```python
from build123d import *

# Parameters (mm, degrees)
F2_SIZE = 1


with BuildPart() as f1:
    # F0 (on Right) → F1 (revolve)
    with BuildSketch(Plane.YZ):
        Polygon((-16, 4.175502), (-20, 4.175502), (-20, -7.824498), (-16, -7.824498), (-16, -1.824498), (0, -1.824498), (0, 0.175502), (-16, 0.175502), align=None)
    revolve(axis=Axis((0, 0, -1.638931), (0, 0, -1)))

    # F2
    f2_edges = [f1.edges().sort_by_distance(p)[0] for p in [
        (0, 16, 4.175502),
        (0, 20, 4.175502),
        (0, 20, -7.824498),
        (0, 16, -7.824498),
    ]]
    chamfer(f2_edges, length=F2_SIZE)


solid = f1.part
```
CAD build for the part. Positions are in the model's coordinates, mm. A direction names the side the tool comes from. Round coordinates to 2 decimals unless told otherwise and drop trailing zeros. Loops run counter-clockwise (first coordinate to the right, second up) from the corner with the lowest first, then second, coordinate; pieces in that order, holes last. Notation, with made-up numbers: M -8.5,-28.5 L -1.5,-28.5 A31 ccw -1.5,3.5 Z; hole C 16,89.25 d5. An arc over 180 degrees is marked long. Return JSON: item names as keys, results as strings. Group by question number.
(1) Tool access for faces 1 (the cylindrical face through (15.62, 3.47, -4.29)), 2 (the flat face through (0, 0, 0.176)), 3 (the flat face through (10, 14, -7.824)): list every direction of +Z, -Z, +X, -X, +Y, -Y with a clear straight run to the whole face (end or side of a thin tool).
(2) Wall check: probe 1 along X at (y, z) = (0, 2.5); probe 2 along Z at (x, y) = (-6.5, 7). Give the ranges that are in metal, low to high. Write a range as [from, to].
(3) Mould opens along X. For faces 4 (the flat face through (10, -14, 4.176)), 5 (the cylindrical face through (19.524, 4.336, -1.894)), 6 (the flat face through (0, 0, -1.824)) say: +X half, -X half, draft (parallel to the pull), parting line (faces both ways), or undercut.
(4) Drop flat-ended pins along their axis: P1, Ø2, axis at y = -1, z = 2.5, coming from the +X side; P2, Ø12, axis at x = -6, y = 13.5, coming from the +Z side; P3, Ø3, axis at x = -6.5, z = -2, coming from the +Y side; P4, Ø3, axis at x = 3.5, z = -0.5, coming from the -Y side. Give the stop position or say it passes through.
(5) Saw through at C-C, the plane z = -5.5. List the corners of the cut face in (x, y), and give its area (3 significant figures).
(6) Saw through at A-A, the plane x = 0. List the corners of the cut face in (y, z), and give its area (3 significant figures).
(7) Saw through at D-D, the plane z = -0.5. List the corners of the cut face in (x, y), and give its area (3 significant figures).
Answer list:
{
 "1": {"face 1": "-Z", "face 2": "+Z", "face 3": "-Z, +X, -X, +Y, -Y"},
 "2": {"probe 1": "[-20, -16], [16, 20]", "probe 2": "[-1.82, 0.18]"},
 "3": {"face 4": "draft", "face 5": "parting line", "face 6": "undercut"},
 "4": {"P1": "x = 20", "P2": "z = 4.18", "P3": "y = 19.36", "P4": "y = -19.9"},
 "5": {"outline": "C 0,0 d40; hole C 0,0 d32", "area": "452 mm2"},
 "6": {"outline": "M -20,-6.82 L -19,-7.82 L -17,-7.82 L -16,-6.82 L -16,-1.82 L 16,-1.82 L 16,-6.82 L 17,-7.82 L 19,-7.82 L 20,-6.82 L 20,3.18 L 19,4.18 L 17,4.18 L 16,3.18 L 16,0.18 L -16,0.18 L -16,3.18 L -17,4.18 L -19,4.18 L -20,3.18 Z", "area": "156 mm2"},
 "7": {"outline": "C 0,0 d40", "area": "1,260 mm2"}
}
